```python
from build123d import *

# Parameters (mm, degrees)
BOSS_EXTRUDE2_DEPTH = 6.75
CUT_EXTRUDE1_DEPTH  = 102.982599985
BOSS_EXTRUDE3_DEPTH = 18
LPATTERN1_COUNT     = 5
LPATTERN1_PITCH     = 5
FILLET1_R           = 8
FILLET2_R           = 5
SKETCH6_R           = 1.5
CUT_EXTRUDE2_DEPTH  = 102.325844179
CUT_EXTRUDE4_DEPTH  = 8
SKETCH9_R           = 1.75
BOSS_EXTRUDE4_DEPTH = 1.5
SKETCH10_R          = 1.75
BOSS_EXTRUDE5_DEPTH = 1.5
CUT_EXTRUDE6_START  = -1.5
CUT_EXTRUDE6_DEPTH  = 103.825844179


with BuildPart() as part:
    # Sketch2 → Boss-Extrude2 (new, symmetric)
    with BuildSketch(Plane(origin=(0, 0, 0), x_dir=(0, 0, -1), z_dir=(1, 0, 0))):
        with BuildLine():
            Line((-2.079082888, 77.410237912), (20.329453697, 7.410237912))
            Line((20.329453697, 7.410237912), (13.081464201, -0.95554047))
            Line((13.081464201, -0.95554047), (13.081464201, -10.95554047))
            Line((13.081464201, -10.95554047), (25.46023991, -14.926171648))
            Line((25.46023991, -14.926171648), (34.052646544, -43.669354287))
            Line((34.052646544, -43.669354287), (34.052646544, -50.669354287))
            Line((34.052646544, -50.669354287), (45.052646544, -50.669354287))
            Line((45.052646544, -50.669354287), (45.052646544, -0.669354287))
            Line((45.052646544, -0.669354287), (51.414117074, 3.570151924))
            Line((51.414117074, 3.570151924), (53.374039372, 4.876312617))
            ThreePointArc((53.374039372, 4.876312617), (53.374039372, 13.361593991), (44.888757997, 13.361593991))
            Line((44.888757997, 13.361593991), (35.302946487, 7.410237912))
            Line((35.302946487, 7.410237912), (28.081464201, 13.727383878))
            Line((28.081464201, 13.727383878), (20.778287365, 84.727383878))
            Line((20.778287365, 84.727383878), (-2.079082888, 77.410237912))
        make_face()
    extrude(amount=BOSS_EXTRUDE2_DEPTH, both=True)

    # Sketch4 → Cut-Extrude1 (cut, through all)
    with BuildSketch(Plane(origin=(6.75, 0, 0), x_dir=(0, 0, -1), z_dir=(1, 0, 0))):
        Polygon((42.352646544, -43.669354287), (42.352646544, -18.669354287), (27.352646544, -18.669354287), align=None)
    extrude(amount=-CUT_EXTRUDE1_DEPTH, mode=Mode.SUBTRACT)

    # Sketch5 → Boss-Extrude3 (add)
    with BuildSketch(Plane(origin=(6.75, 0, 0), x_dir=(0, 0, -1), z_dir=(1, 0, 0))):
        Polygon((49.052646544, -43.669354287), (45.052646544, -41.669354287), (45.052646544, -43.669354287), align=None)
        Polygon((49.052646544, -43.669354287), (45.052646544, -43.669354287), (45.052646544, -45.669354287), align=None)
    boss_extrude3 = extrude(amount=-BOSS_EXTRUDE3_DEPTH)

    # LPattern1: Boss-Extrude3 ×5
    with Locations(*[(0, i * LPATTERN1_PITCH, 0) for i in range(1, LPATTERN1_COUNT)]):
        add(boss_extrude3)

    # Fillet1
    fillet1_edges = [part.edges().sort_by_distance(p)[0] for p in [
        (0, -10.95554047, -13.081464201),
        (0, -0.95554047, -13.081464201),
    ]]
    fillet(fillet1_edges, radius=FILLET1_R)

    # Fillet2
    fillet2_edges = [part.edges().sort_by_distance(p)[0] for p in [
        (0, 77.410237912, 2.079082888),
        (0, 84.727383878, -20.778287365),
    ]]
    fillet(fillet2_edges, radius=FILLET2_R)

    # Sketch6 → Cut-Extrude2 (cut, through all)
    with BuildSketch(Plane(origin=(6.75, 0, 0), x_dir=(0, 0, -1), z_dir=(1, 0, 0))):
        with Locations((4.207274657, 74.172691185)):
            Circle(SKETCH6_R)
    extrude(amount=-CUT_EXTRUDE2_DEPTH, mode=Mode.SUBTRACT)

    # Sketch8 → Cut-Extrude4 (cut)
    with BuildSketch(Plane(origin=(0, 5.762226271, -19.275708093), x_dir=(1, 0, 0), z_dir=(0, -0.28641355449068423, 0.9581060879693918))):
        Polygon((-3.75, -30.834539791), (3.75, -30.834539791), (9.054771206, -45.201974161), (-2.945228794, -45.201974161), align=None)
    extrude(amount=-CUT_EXTRUDE4_DEPTH, mode=Mode.SUBTRACT)

    # Sketch9 → Boss-Extrude4 (add)
    with BuildSketch(Plane(origin=(6.75, 0, 0), x_dir=(0, 0, -1), z_dir=(1, 0, 0))):
        with Locations((49.131398685, 9.118953304)):
            Circle(SKETCH9_R)
    boss_extrude4 = extrude(amount=BOSS_EXTRUDE4_DEPTH)

    # Sketch10 → Boss-Extrude5 (add)
    with BuildSketch(Plane(origin=(6.75, 0, 0), x_dir=(0, 0, -1), z_dir=(1, 0, 0))):
        with Locations((21.081464201, -5.120153169)):
            Circle(SKETCH10_R)
    boss_extrude5 = extrude(amount=BOSS_EXTRUDE5_DEPTH)

    # Sketch11 → Cut-Extrude6 (cut)
    with BuildSketch(Plane(origin=(6.75, 0, 0), x_dir=(0, 0, -1), z_dir=(1, 0, 0)).offset(CUT_EXTRUDE6_START)):
        with BuildLine():
            Line((15.78419602, 72.628770071), (6.886860744, 69.780537742))
            ThreePointArc((6.886860744, 69.780537742), (6.316756639, 69.312297005), (6.22287904, 68.580549047))
            Line((6.22287904, 68.580549047), (7.115164558, 65.08899702))
            Line((7.115164558, 65.08899702), (18.222367047, 30.392212101))
            ThreePointArc((18.222367047, 30.392212101), (19.230775138, 29.698663405), (20.155274557, 30.50065935))
            Line((20.155274557, 30.50065935), (20.931307176, 34.374295724))
            Line((20.931307176, 34.374295724), (17.083828456, 71.778701405))
            ThreePointArc((17.083828456, 71.778701405), (16.636465842, 72.51325811), (15.78419602, 72.628770071))
        make_face()
    cut_extrude6 = extrude(amount=CUT_EXTRUDE6_DEPTH, mode=Mode.SUBTRACT)

    # Mirror1: Boss-Extrude4, Boss-Extrude5, Cut-Extrude6 across plane
    add(boss_extrude4.mirror(Plane(origin=(0, 0, 0), x_dir=(0, 0, 1), z_dir=(1, 0, 0))))
    add(boss_extrude5.mirror(Plane(origin=(0, 0, 0), x_dir=(0, 0, 1), z_dir=(1, 0, 0))))
    add(cut_extrude6.mirror(Plane(origin=(0, 0, 0), x_dir=(0, 0, 1), z_dir=(1, 0, 0))), mode=Mode.SUBTRACT)


solid = part.part
```
Read the model definition and answer for the solid it produces. Units are mm, in the model's axes. A direction names the side the tool comes from. Give positions to 0.01 mm unless a question says otherwise; leave off trailing zeros. Write each loop counter-clockwise with the first axis right and the second up, starting at its lowest first coordinate (ties: lowest second). Pieces come first, ordered by that corner, then holes. Notation, with made-up numbers: (19, 62.25) -> (39, 62.25) arc R21 ccw to (39, 84.25) -> close; hole circle Ø5 at (83, 34). An arc over 180 degrees is marked (long way). Answer as a JSON object with one key per item and string values.
1) For a pull along Z with two mould halves and no side action, classify faces 4 (the flat face through (-9, -34, -45.053)), 5 (the flat face through (-2.124, -22.683, -47.081)), 6 (the flat face through (5.99, 71.225, -11.398)) as pulls with the +Z half, pulls with the -Z half, needs draft (parallel to the pull), parting line crosses it, or undercut.
Findings below:
{"face 4": "pulls with the +Z half", "face 5": "pulls with the -Z half", "face 6": "undercut"}
2) A tool of negligible diameter and unlimited length cuts with its end or side. For faces 1 (the flat face through (-2.124, -37.683, -47.081)), 2 (the flat face through (1.97, -36.74, -34.92)), 3 (the flat face through (0.095, 10.525, -31.743)), from which of +Z, -Z, +X, -X, +Y, -Y can it reach the whole face along a straight path? Write none if from no direction.
Findings below:
{"face 1": "-Z, +X, -X", "face 2": "+Z, +X", "face 3": "+X, -X, +Y"}
3) Flat-ended cylindrical pins translate along their axes: pin 1 Ø8 at (x, y) = (1, 69.5) entering from +Z; pin 2 Ø7.5 at (y, z) = (40.5, -14) entering from -X; pin 3 Ø1.2 at (x, y) = (-10, -34.5) entering from +Z. Find the tip coordinate at first contact, or state that the pin passes through.
Findings below:
{"pin 1": "stops at z = 0.75", "pin 2": "stops at x = -6.75", "pin 3": "stops at z = -45.05"}
4) Straight lines are drawn through the part: probe 1 along Y at (x, z) = (-2, -48); probe 2 along X at (y, z) = (-5, -24); probe 3 along Z at (x, y) = (-4.75, -20.5). For each, find the intervals that lie inside material, in ascending order. Write a range as from..to.
Findings below:
{"probe 1": "y = -44.2..-43.14, -39.2..-38.14, -34.2..-33.14, -29.2..-28.14, -24.2..-23.14, 1.29..15.01", "probe 2": "x = -6.75..6.75", "probe 3": "z = -45.05..-42.35, -28.45..-27.13"}
5) Section A-A on y = 47.5 is taken. Write down the section's boundary in (x, z).
Findings below:
{"outline": "(-6.75, -24.61) -> (6.75, -24.61) -> (6.75, -19.58) -> (5.25, -19.58) -> (5.25, -12.75) -> (6.75, -12.75) -> (6.75, -7.5) -> (-6.75, -7.5) -> (-6.75, -12.75) -> (-5.25, -12.75) -> (-5.25, -19.58) -> (-6.75, -19.58) -> close"}
